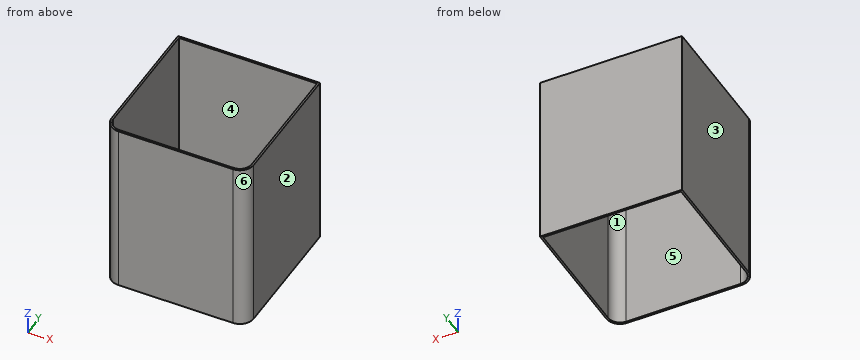
```python
from build123d import *

# Parameters (mm, degrees)
BOSS_EXTRUDE1_DEPTH = 180


with BuildPart() as part:
    # Sketch1 → Boss-Extrude1 (new body)
    with BuildSketch(Plane.XY):
        with BuildLine():
            Line((-58, -72), (58, -72))
            ThreePointArc((58, -72), (67.899494937, -67.899494937), (72, -58))
            Line((72, -58), (72, 72))
            Line((72, 72), (-72, 72))
            Line((-72, 72), (-72, -58))
            ThreePointArc((-72, -58), (-67.899494937, -67.899494937), (-58, -72))
        make_face()
        with BuildLine():
            Line((-70, -58), (-70, 70))
            Line((-70, 70), (70, 70))
            Line((70, 70), (70, -58))
            ThreePointArc((70, -58), (66.485281374, -66.485281374), (58, -70))
            Line((58, -70), (-58, -70))
            ThreePointArc((-58, -70), (-66.485281374, -66.485281374), (-70, -58))
        make_face(mode=Mode.SUBTRACT)
    extrude(amount=BOSS_EXTRUDE1_DEPTH)


solid = part.part
```
The model under review builds one solid part; all positions refer to its coordinate system, in mm. Face numbers are marked on the shaded views. A direction names the side the tool comes from. Round coordinates to 2 decimals unless told otherwise and drop trailing zeros. Loops run counter-clockwise (first coordinate to the right, second up) from the corner with the lowest first, then second, coordinate; pieces in that order, holes last. Notation, with made-up numbers: (22, 30.5) - (64, 30.5) arc R12 ccw to (64, 36.5) - close; hole circle Ø5 at (89.5, 51). An arc over 180 degrees is marked (long way). Use a Markdown table: item, result. Add a question column.
Q1. For probe 1 along Y at (x, z) = (-7, 28); probe 2 along Y at (x, z) = (-60, 111), list the stretches that pass through material, from the lowest coordinate up.
Q2. The part is to be moulded in two halves that separate along X. For the marked faces 3, 4, 5 and 6, say which applies: pulls with the +X half, pulls with the -X half, needs draft (parallel to the pull), parting line crosses it, or undercut.
Q3. Machinability: for the marked faces 1 and 2, which of the approach directions +Z, -Z, +X, -X, +Y, -Y give a long, thin tool a straight path to every point of the face, cutting with its end or side? Answer none if there is none.
Q4. Add section A-A (x = 43). State the section outline as (y, z) points, plus the area to 3 significant figures.
Q5. Add section B-B (z = 54). State the section outline as (x, y) points, plus the area to 3 significant figures.
Worked answers:
| question | item | result |
|---|---|---|
| 1 | probe 1 | -72 to -70, 70 to 72 |
| 1 | probe 2 | -71.86 to -69.83, 70 to 72 |
| 2 | face 3 | pulls with the -X half |
| 2 | face 4 | undercut |
| 2 | face 5 | undercut |
| 2 | face 6 | pulls with the +X half |
| 3 | face 1 | +Z, -Z |
| 3 | face 2 | +Z, -Z, +X, +Y, -Y |
| 4 | outline | (-72, 0) - (-70, 0) - (-70, 180) - (-72, 180) - close; (70, 0) - (72, 0) - (72, 180) - (70, 180) - close |
| 4 | area | 720 mm² |
| 5 | outline | (-72, -58) arc R14 ccw to (-58, -72) - (58, -72) arc R14 ccw to (72, -58) - (72, 72) - (-72, 72) - close; hole (-70, -58) arc R12 ccw to (-58, -70) - (58, -70) arc R12 ccw to (70, -58) - (70, 70) - (-70, 70) - close |
| 5 | area | 1,110 mm² |
